Can you work these out from the model? Positions are in its coordinate system, mm. Round coordinates to 2 decimals unless told otherwise and drop trailing zeros. Order: outer loops, then holes, each group sorted by start corner. A loop starts at its lowest first (then second) coordinate and runs counter-clockwise, first axis right, second up.
Q1. If we section it at C-C (z = 1): Count the separate pieces of the cut face and the enclosed holes in it, plus the area to 3 significant figures.
Q2. If we section it at D-D (x = 17): Please give me the cut outline in (y, z).
Q3. If I drill on line 1 (Y direction, x = 0, z = 4); line 2 (Y direction, x = 0, z = 2.5); line 3 (X direction, y = 32, z = 3.75), over which ranges is the centre line in solid material (lowest first)?
Q4. Will these pins go through, and if not, where does the flat tip stop? P1, Ø7, axis at x = 0, y = 32, coming from the +Z side; P2, Ø3, axis at x = -4, z = 4.5, coming from the -Y side; P3, Ø3, axis at y = 19.5, z = 5, coming from the +X side; P4, Ø2, axis at x = -4, z = 5, coming from the +Y side.
Q5. If we section it at A-A (x = -32): Please give me the cut outline in (y, z).
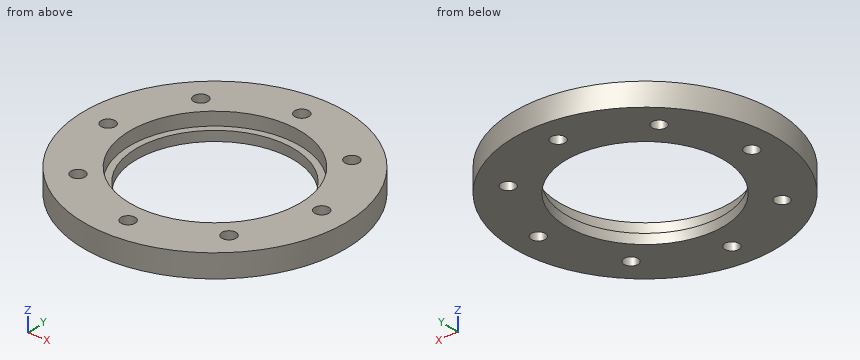
Autodesk Inventor part; units mm, degrees
ref_plane "YZ Plane" through (0, 0, 0) normal (1, 0, 0) x (0, 1, 0)
ref_plane "XZ Plane" through (0, 0, 0) normal (0, 1, 0) x (-1, 0, 0)
ref_plane "XY Plane" through (0, 0, 0) normal (0, 0, 1) x (1, 0, 0)
sketch "スケッチ1" plane through (0, 0, 0) normal (1, 0, 0) x (0, 1, 0)
  line L0 (24, 0) -> (40, 0)
  line L1 (40, 0) -> (40, 7)
  line L2 (40, 7) -> (26, 7)
  line L3 (26, 7) -> (26, 3)
  line L4 (26, 3) -> (24, 3)
  line L5 (24, 3) -> (24, 0)
  line L6 (0, -1.4) -> (0, 8.4)
  point P0 (0, 0)
  dimension "d0" = 24
  dimension "d1" = 40
  dimension "d2" = 26
  dimension "d3" = 4
  dimension "d5" = 3
revolve "回転1" add sketch "スケッチ1" angle 360 about axis through (0, 0, -10) along (0, 0, 1)
sketch "スケッチ2" plane through (0, 0, 7) normal (0, 0, 1) x (1, 0, 0)
  circle A0 centre (0, 0) radius 32
  point P0 (0, 32)
  point P1 (-22.6274, 22.6274)
  point P2 (-32, 0)
  point P3 (-22.6274, -22.6274)
  point P4 (0, -32)
  point P5 (22.6274, -22.6274)
  point P6 (32, 0)
  point P7 (22.6274, 22.6274)
  dimension "d7" = 64
  dimension "d10" = 360
hole "穴1" at (0, 32, 7) at (-22.6274, 22.6274, 7) at (-32, 0, 7) at (-22.6274, -22.6274, 7) at (0, -32, 7) at (22.6274, -22.6274, 7) at (32, 0, 7) at (22.6274, 22.6274, 7) direction (0, 0, -1) diameter 4.3 end through all
properties part number "base8" material "ABS プラスチック"
Solution:
1. separate pieces: 1
1. enclosed holes: 9
1. area: 3,100 mm2
2. outline: (-36.21, 0) - (-16.94, 0) - (-16.94, 3) - (-19.67, 3) - (-19.67, 7) - (-36.21, 7) - close; (16.94, 0) - (36.21, 0) - (36.21, 7) - (19.67, 7) - (19.67, 3) - (16.94, 3) - close
3. line 1: y = -40 to -34.15, -29.85 to -26, 26 to 29.85, 34.15 to 40
3. line 2: y = -40 to -34.15, -29.85 to -24, 24 to 29.85, 34.15 to 40
3. line 3: x = -24 to -2.15, 2.15 to 24
4. P1: stops at z = 7
4. P2: stops at y = -39.92
4. P3: stops at x = 35.72
4. P4: stops at y = 39.89
5. outline: (-24, 0) - (-2.15, 0) - (-2.15, 7) - (-24, 7) - close; (2.15, 0) - (24, 0) - (24, 7) - (2.15, 7) - close
